The drawing under review shows one solid part. Ordinate dimensions are in mm from its lowest x, y, z. A direction names the side the tool comes from. Coordinates: 2 decimals unless noted, no trailing zeros. Loops run counter-clockwise (first coordinate to the right, second up) from the corner with the lowest first, then second, coordinate; pieces in that order, holes last. Notation, with made-up numbers: M 48,64 L 95,64 A13 cw 95,88 Z; hole C 55.25,-6.5 d6. An arc over 180 degrees is marked long. Use one line per item in the form item = value.
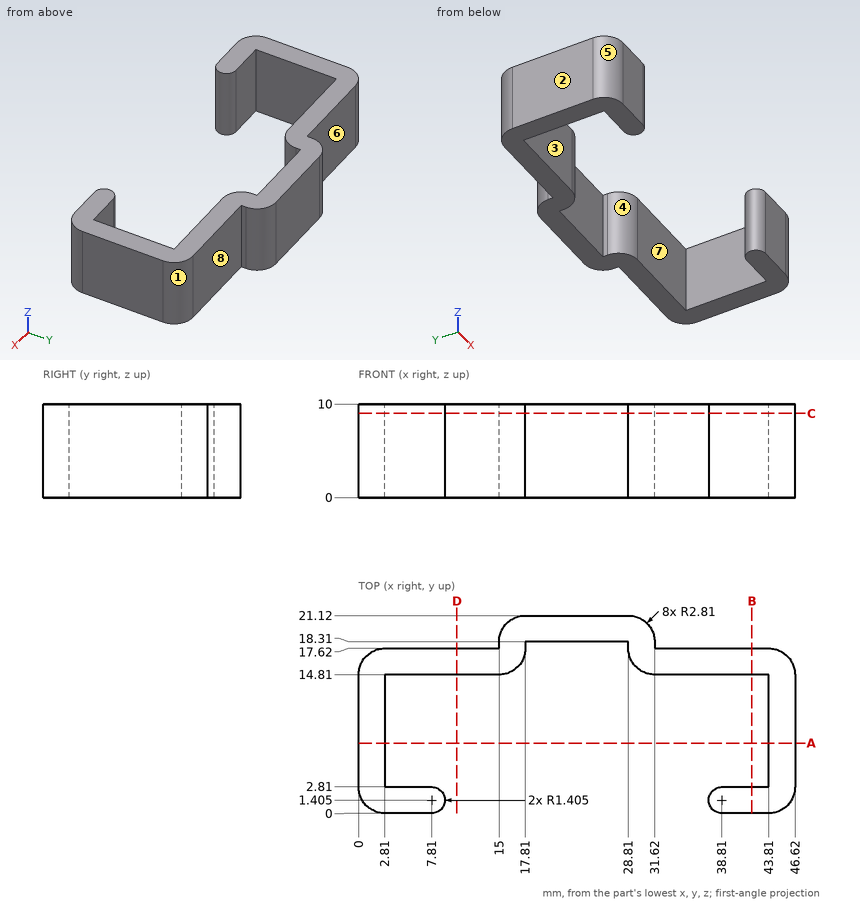
1. Consider section B-B on x = 42. Write out the cut boundary in (y, z).
Computed values:
outline = M 0,0 L 2.81,0 L 2.81,10 L 0,10 Z; M 14.81,0 L 17.62,0 L 17.62,10 L 14.81,10 Z
2. Consider section C-C on z = 9. Write out the cut boundary in (x, y) (3 decimals), plus the area to 3 significant figures.
Computed values:
outline = M 0,2.81 A2.81 ccw 2.81,0 L 7.81,0 A1.405 ccw 7.81,2.81 L 2.81,2.81 L 2.81,14.81 L 15,14.81 A2.81 ccw 17.81,17.62 L 17.81,18.31 L 28.81,18.31 L 28.81,17.62 A2.81 ccw 31.62,14.81 L 43.81,14.81 L 43.81,2.81 L 38.81,2.81 A1.405 ccw 38.81,0 L 43.81,0 A2.81 ccw 46.62,2.81 L 46.62,14.81 A2.81 ccw 43.81,17.62 L 31.62,17.62 L 31.62,18.31 A2.81 ccw 28.81,21.12 L 17.81,21.12 A2.81 ccw 15,18.31 L 15,17.62 L 2.81,17.62 A2.81 ccw 0,14.81 Z
area = 255 mm2
3. For pin 1 Ø1.5 at (x, z) = (6.5, 5.5) entering from +Y; pin 2 Ø0.6 at (y, z) = (18, 5) entering from +X; pin 3 Ø3 at (x, z) = (9.5, 6.5) entering from -Y, all flat-tipped, find the tip position at first contact; note any pin that passes through.
Computed values:
pin_1 = 17.62
pin_2 = 31.62
pin_3 = 0.01
4. Wall thickness on line 1 along X through (y, z) = (3.5, 7); line 2 along Y through (x, z) = (6.5, 6.75); line 3 along Y through (x, z) = (36, 2.5): over which ranges is each line inside the solid? List them lowest first. Write a range as from..to.
Computed values:
line_1 = 0..2.81, 43.81..46.62
line_2 = 0..2.81, 14.81..17.62
line_3 = 14.81..17.62
5. Consider section A-A on y = 7.5. Write out the cut boundary in (x, z).
Computed values:
outline = M 0,0 L 2.81,0 L 2.81,10 L 0,10 Z; M 43.81,0 L 46.62,0 L 46.62,10 L 43.81,10 Z
6. Draft analysis for pull direction X (two halves, no side actions). For the marked faces 1, 2 and 3, state which applies: +X half, -X half, draft (parallel to the pull), parting line (faces both ways), or undercut.
Computed values:
face_1 = +X half
face_2 = -X half
face_3 = undercut
7. Consider section D-D on x = 10.5. Write out the cut boundary in (y, z), plus the area to 3 significant figures.
Computed values:
outline = M 14.81,0 L 17.62,0 L 17.62,10 L 14.81,10 Z
area = 28.1 mm2
8. Tool access review of the marked faces 4, 5, 6, 7 and 8: name each direction out of +Z, -Z, +X, -X, +Y, -Y from which nothing blocks a thin tool from reaching the whole face with its end or side.
Computed values:
face_4 = +Z, -Z, -Y
face_5 = +Z, -Z, -X, -Y
face_6 = +Z, -Z, -X, +Y
face_7 = +Z, -Z
face_8 = +Z, -Z, +X, +Y
